Read the model definition and answer for the solid it produces. Units are mm, in the model's axes. A direction names the side the tool comes from. Coordinates: 2 decimals unless noted, no trailing zeros. Loops run counter-clockwise (first coordinate to the right, second up) from the corner with the lowest first, then second, coordinate; pieces in that order, holes last.
from build123d import *

# Parameters (mm, degrees)
SKETCH1_R           = 2.1
SKETCH1_R_2         = 2
SKETCH1_W           = 7
SKETCH1_H           = 2
BOSS_EXTRUDE1_DEPTH = 5


with BuildPart() as part:
    # Sketch1 → Boss-Extrude1 (new body)
    with BuildSketch(Plane.XY):
        Polygon((0, 0), (0, 82), (-80, 82), (-80, 67), (-20.191582532, 40), (-20.191582532, 0), align=None)
        with Locations((-10.095791266, 10)):
            Circle(SKETCH1_R, mode=Mode.SUBTRACT)
        with Locations((-10.095791266, 30)):
            Circle(SKETCH1_R, mode=Mode.SUBTRACT)
        with Locations((-70, 74.5)):
            Circle(SKETCH1_R_2, mode=Mode.SUBTRACT)
        with Locations((-50, 74.5)):
            Circle(SKETCH1_R_2, mode=Mode.SUBTRACT)
        with Locations((-30, 74.5)):
            Circle(SKETCH1_R_2, mode=Mode.SUBTRACT)
        with Locations((-10, 74.5)):
            Circle(SKETCH1_R_2, mode=Mode.SUBTRACT)
        with Locations((-10.095791266, 4)):
            Rectangle(SKETCH1_W, SKETCH1_H, mode=Mode.SUBTRACT)
    extrude(amount=BOSS_EXTRUDE1_DEPTH)


solid = part.part
Item 1: Find the intervals of material crossed by line 1 along Y through (x, z) = (-11, 3.6); line 2 along Y through (x, z) = (-50, 3.15); line 3 along Y through (x, z) = (-10.5, 1.15), in increasing order.
Numbers:
line 1: y = 0 to 3, 5 to 8.1, 11.9 to 28.1, 31.9 to 72.77, 76.23 to 82
line 2: y = 53.46 to 72.5, 76.5 to 82
line 3: y = 0 to 3, 5 to 7.94, 12.06 to 27.94, 32.06 to 72.56, 76.44 to 82
Item 2: A cutting plane is placed at D-D on x = -10. Determine the outline of the cut face in (y, z), then the cut area to 3 significant figures.
Numbers:
outline: (0, 0) - (3, 0) - (3, 5) - (0, 5) - close; (5, 0) - (7.9, 0) - (7.9, 5) - (5, 5) - close; (12.1, 0) - (27.9, 0) - (27.9, 5) - (12.1, 5) - close; (32.1, 0) - (72.5, 0) - (72.5, 5) - (32.1, 5) - close; (76.5, 0) - (82, 0) - (82, 5) - (76.5, 5) - close
area: 338 mm2
Item 3: A cutting plane is placed at B-B on z = 1.6. Determine the outline of the cut face in (x, y).
Numbers:
outline: (-80, 67) - (-20.19, 40) - (-20.19, 0) - (0, 0) - (0, 82) - (-80, 82) - close; hole circle Ø4 at (-70, 74.5); hole circle Ø4 at (-50, 74.5); hole circle Ø4 at (-30, 74.5); hole (-13.6, 3) - (-6.6, 3) - (-6.6, 5) - (-13.6, 5) - close; hole circle Ø4.2 at (-10.1, 10); hole circle Ø4.2 at (-10.1, 30); hole circle Ø4 at (-10, 74.5)
Item 4: Determine the mould class of faces 4 (the face through (-68.925, 76.186, 2.465)), 5 (the face through (-11.644, 11.419, 2.465)), 6 (the face through (0, 40, 2)), 7 (the face through (-50.514, 53.689, 2.465)) for opening direction X: released by +X, released by -X, zero draft, split by the parting line, or undercut.
Numbers:
face 4: undercut
face 5: undercut
face 6: released by +X
face 7: released by -X
Item 5: A cutting plane is placed at A-A on y = 74.5. Determine the outline of the cut face in (x, z), then the cut area to 3 significant figures.
Numbers:
outline: (-80, 0) - (-72, 0) - (-72, 5) - (-80, 5) - close; (-68, 0) - (-52, 0) - (-52, 5) - (-68, 5) - close; (-48, 0) - (-32, 0) - (-32, 5) - (-48, 5) - close; (-28, 0) - (-12, 0) - (-12, 5) - (-28, 5) - close; (-8, 0) - (0, 0) - (0, 5) - (-8, 5) - close
area: 320 mm2
Item 6: Given pin 1 (3.5 mm diameter, centred on x = -70, y = 74.5, fed in from -Z); pin 2 (1.5 mm diameter, centred on y = 13.5, z = 3.5, fed in from -X), each flat-ended and moving along its own axis, determine where each tip first touches the part or whether it passes through.
Numbers:
pin 1: passes through
pin 2: stops at x = -20.19
Item 7: Which of the six approach directions +Z, -Z, +X, -X, +Y, -Y give full straight-line access (tool end or side, diameter ignored) to faces 1 (the face through (-32, 60, 0)), 2 (the face through (-20.192, 20, 2)), 3 (the face through (-6.596, 4, 2))?
Numbers:
face 1: -Z, +X, -X, +Y, -Y
face 2: +Z, -Z, -X, -Y
face 3: +Z, -Z
Item 8: A cutting plane is placed at C-C on x = -50. Determine the outline of the cut face in (y, z), then the cut area to 3 significant figures.
Numbers:
outline: (53.46, 0) - (72.5, 0) - (72.5, 5) - (53.46, 5) - close; (76.5, 0) - (82, 0) - (82, 5) - (76.5, 5) - close
area: 123 mm2
